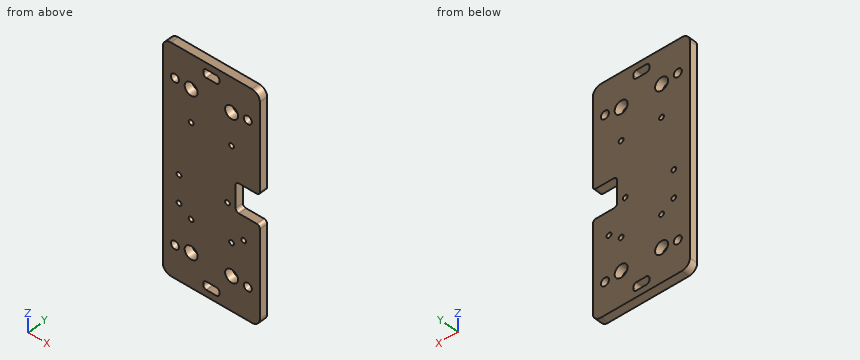
Autodesk Inventor part; units mm, degrees
ref_plane "YZ Plane" through (0, 0, 0) normal (1, 0, 0) x (0, 1, 0)
ref_plane "XZ Plane" through (0, 0, 0) normal (0, 1, 0) x (-1, 0, 0)
ref_plane "XY Plane" through (0, 0, 0) normal (0, 0, 1) x (1, 0, 0)
sketch "Sketch1" plane through (0, 0, 0) normal (0, 1, 0) x (-1, 0, 0)
  line L0 (0, 0) -> (60, 0)
  line L1 (60, 0) -> (60, -140)
  line L2 (60, -140) -> (0, -140)
  line L3 (0, -140) -> (0, 0)
  line L4 (30, -20.8594) -> (30, -183.1932) construction
  line L5 (42.5, -21.7206) -> (42.5, -191.0157) construction
  line L6 (17.5, -21.7206) -> (17.5, -184.1979) construction
  circle A0 centre (42.5, -21) radius 4
  circle A1 centre (42.5, -41) radius 1.5
  circle A2 centre (42.5, -99) radius 1.5
  circle A3 centre (42.5, -119) radius 4
  circle A4 centre (17.5, -99) radius 1.5
  circle A5 centre (17.5, -119) radius 4
  circle A6 centre (17.5, -41) radius 1.5
  circle A7 centre (17.5, -21) radius 4
  dimension "d0" = 140
  dimension "d1" = 60
  dimension "d2" = 30
  dimension "d3" = 12.5
  dimension "d4" = 12.5
  dimension "d5" = 8
  dimension "d6" = 3
  dimension "d7" = 3
  dimension "d8" = 8
  dimension "d9" = 3
  dimension "d10" = 8
  dimension "d11" = 3
  dimension "d13" = 20
  dimension "d14" = 20
  dimension "d15" = 20
  dimension "d16" = 20
  dimension "d17" = 21
  dimension "d18" = 21
  dimension "d19" = 21
  dimension "d20" = 21
  dimension "d74" = 8
extrude "Extrusion1" add sketch "Sketch1" along normal blind 5
sketch "Sketch2" plane through (0, 0, 0) normal (0, -1, 0) x (1, 0, 0)
  circle A0 centre (-7.5, -20) radius 2.5
  circle A1 centre (-7.5, -120) radius 2.5
  circle A2 centre (-52.5, -20) radius 2.5
  circle A3 centre (-52.5, -120) radius 2.5
  line L0 (-60, 0) -> (0, 0)
  line L1 (0, 0) -> (0, -140)
  line L2 (-60, -140) -> (-60, 0)
  line L3 (0, -140) -> (-60, -140)
  dimension "d23" = 5
  dimension "d24" = 5
  dimension "d25" = 5
  dimension "d26" = 5
  dimension "d27" = 20
  dimension "d28" = 7.5
  dimension "d29" = 20
  dimension "d30" = 7.5
  dimension "d31" = 20
  dimension "d32" = 7.5
  dimension "d33" = 20
  dimension "d34" = 7.5
extrude "Extrusion2" cut sketch "Sketch2" against normal blind 10 contours A0 | A1 | A2 | A3
sketch "Sketch3" plane through (0, 0, 0) normal (0, -1, 0) x (1, 0, 0)
  line L0 (-25, -4) -> (-35, -4)
  line L1 (-35, -4) -> (-35, -9)
  line L2 (-35, -9) -> (-25, -9)
  line L3 (-25, -9) -> (-25, -4)
  line L4 (9.3646, -70) -> (-76.8402, -70) construction
  line L5 (-60, 0) -> (0, 0)
  line L6 (0, 0) -> (0, -140)
  line L7 (-25, -136) -> (-35, -136)
  line L8 (-35, -136) -> (-35, -131)
  line L9 (-35, -131) -> (-25, -131)
  line L10 (-25, -131) -> (-25, -136)
  dimension "d40" = 70
  dimension "d41" = 10
  dimension "d42" = 4
  dimension "d43" = 5
  dimension "d44" = 25
extrude "Extrusion3" cut sketch "Sketch3" against normal blind 10
fillet "Fillet2" radius 5 4 edges at (-60, 2.5, 0) (-60, 2.5, -140) (0, 2.5, -140) (0, 2.5, 0)
sketch "Sketch4" plane through (0, 5, 0) normal (0, 1, 0) x (1, 0, 0)
  circle A0 centre (-50, 76.5) radius 1.5
  circle A1 centre (-50, 93.5) radius 1.5
  circle A2 centre (-20, 76.5) radius 1.5
  circle A3 centre (-10, 93.5) radius 1.5
  line L0 (-5, 140) -> (-55, 140)
  line L1 (-60, 135) -> (-60, 5)
  line L2 (0, 5) -> (0, 135)
  point P0 (0, 0)
  dimension "d49" = 3
  dimension "d50" = 3
  dimension "d51" = 3
  dimension "d52" = 3
  dimension "d53" = 46.5
  dimension "d54" = 46.5
  dimension "d55" = 63.5
  dimension "d56" = 63.5
  dimension "d57" = 10
  dimension "d59" = 10
  dimension "d71" = 10
  dimension "d72" = 20
extrude "Extrusion4" cut sketch "Sketch4" against normal blind 10
sketch "Sketch5" plane through (0, 0, 0) normal (0, -1, 0) x (1, 0, 0)
  line L0 (59.7124, -61) -> (87.7124, -61)
  line L1 (87.7124, -79) -> (59.7124, -79)
  line L2 (5, -61) -> (-15, -61)
  line L3 (-15, -61) -> (-15, -79)
  line L4 (-15, -79) -> (5, -79)
  line L5 (5, -79) -> (5, -61)
  line L6 (0, -5) -> (0, -135)
  point P0 (0, 0)
  dimension "d66" = 15
  dimension "d67" = 5
extrude "Extrusion5" cut sketch "Sketch5" against normal blind 10
fillet "Fillet3" radius 2 4 edges at (0, 2.5, -79) (0, 2.5, -61) (-15, 2.5, -79) (-15, 2.5, -61)
fillet "Fillet4" radius 2 8 edges at (-25, 2.5, -9) (-25, 2.5, -4) (-35, 2.5, -4) (-35, 2.5, -9) (-35, 2.5, -136) (-35, 2.5, -131) (-25, 2.5, -131) (-25, 2.5, -136)
equation "\"d2\" = 0.5 * d1"
equation "\"d4\" = d3"
equation "\"d8\" = d5"
equation "\"d10\" = d5"
equation "\"d14\" = d13"
equation "\"d15\" = d13"
equation "\"d16\" = d13"
equation "\"d18\" = d17"
equation "\"d19\" = d17"
equation "\"d20\" = d17"
equation "\"d29\" = d27"
equation "\"d30\" = d28"
equation "\"d31\" = d27"
equation "\"d32\" = d28"
equation "\"d33\" = d27"
equation "\"d34\" = d28"
equation "\"d50\" = d49"
equation "\"d51\" = d49"
equation "\"d52\" = d49"
properties part number "Y-Axis_front_plate_top"
Build history of the part. All positions in model axes, mm. Give positions to 0.01 mm unless a question says otherwise; leave off trailing zeros. Loops run counter-clockwise (first coordinate to the right, second up) from the corner with the lowest first, then second, coordinate; pieces in that order, holes last. Notation, with made-up numbers: (-18, 58) -> (3, 58) arc R20 cw to (3, 92) -> close; hole circle Ø2 at (20, 6). An arc over 180 degrees is marked (long way). One line per question, with ' | ' between items. Start each with the question number.
1) Cut at B-B (y = 0.9). Count the separate pieces of the cut face and the enclosed holes in it, plus the area to 3 significant figures.
2) Pin check, flat tip, straight feed: pin 1 (1.5 mm diameter, centred on y = 1.5, z = -67.5, fed in from +X). Stop position of the tip, or through.
3) Probe L1, parallel to Z at x = -30.5, y = 2.5; L2, parallel to Z at x = -18, y = 3.95; L3, parallel to Z at x = -21, y = 2.4. List the from-to ranges inside material, lowest first.
4) Cut at A-A (z = -41). Give the cut face in (x, y), plus the area to 3 significant figures.
Return value:
1) separate pieces: 1 | enclosed holes: 18 | area: 7,680 mm^2
2) pin 1: x = -15
3) L1: -140 to -136, -131 to -9, -4 to 0 | L2: -140 to -122.97, -115.03 to -100.41, -97.59 to -42.41, -39.59 to -24.97, -17.03 to 0 | L3: -140 to -120.94, -117.06 to -77.62, -75.38 to -22.94, -19.06 to 0
4) outline: (-60, 0) -> (-44, 0) -> (-44, 5) -> (-60, 5) -> close; (-41, 0) -> (-19, 0) -> (-19, 5) -> (-41, 5) -> close; (-16, 0) -> (0, 0) -> (0, 5) -> (-16, 5) -> close | area: 270 mm^2
